```python
from build123d import *

# Parameters (mm, degrees)
EXTRUDE_1_DEPTH     = 45
SKETCH_2_W          = 70
SKETCH_2_H          = 80
EXTRUDE_2_DEPTH     = 30
SKETCH_3_W          = 70
SKETCH_3_H          = 60
CUT_EXTRUDE_1_DEPTH = 20
SKETCH_4_W          = 10
SKETCH_4_H          = 20
EXTRUDE_4_DEPTH     = 48
CUT_EXTRUDE_2_DEPTH = 125.222582488
CUT_EXTRUDE_3_DEPTH = 118.153745139


with BuildPart() as part:
    # 草圖1 → 填料-伸長1 (new body)
    with BuildSketch(Plane.XY):
        with BuildLine():
            Line((-15, 0), (-55, 0))
            Line((-55, 0), (-55, -10))
            Line((-55, -10), (-10, -10))
            Line((-10, -10), (-10, 0))
            ThreePointArc((-10, 0), (0, 10), (10, 0))
            Line((10, 0), (10, -10))
            Line((10, -10), (15, -10))
            Line((15, -10), (15, 0))
            ThreePointArc((15, 0), (0, 15), (-15, 0))
        make_face()
    extrude(amount=-EXTRUDE_1_DEPTH)

    # 草圖2 → 填料-伸長2 (add)
    with BuildSketch(Plane.ZY.offset(55)):
        with Locations((-22.5, 30)):
            Rectangle(SKETCH_2_W, SKETCH_2_H)
    extrude(amount=EXTRUDE_2_DEPTH)

    # 草圖3 → 除料-伸長1 (cut)
    with BuildSketch(Plane.ZY.offset(85)):
        with Locations((-22.5, 20)):
            Rectangle(SKETCH_3_W, SKETCH_3_H)
    extrude(amount=-CUT_EXTRUDE_1_DEPTH, mode=Mode.SUBTRACT)

    # 草圖4 → 填料-伸長4 (add)
    with BuildSketch(Plane(origin=(-55, 0, 0), x_dir=(0, 0, -1), z_dir=(1, 0, 0))):
        with Locations((22.5, 10)):
            Rectangle(SKETCH_4_W, SKETCH_4_H)
    extrude(amount=EXTRUDE_4_DEPTH)

    # 草圖6 → 除料-伸長2 (cut, through all)
    with BuildSketch(Plane.XY):
        with BuildLine():
            Line((10, 0), (10, -10))
            Line((10, -10), (-10, -10))
            Line((-10, -10), (-10, 0))
            ThreePointArc((-10, 0), (0, 10), (10, 0))
        make_face()
    extrude(amount=-CUT_EXTRUDE_2_DEPTH, mode=Mode.SUBTRACT)

    # 草圖7 → 除料-伸長3 (cut, through all)
    with BuildSketch(Plane.XY.offset(-17.5)):
        Polygon((-7, 13.266499161), (-55, 20), (-7, 20), align=None)
    extrude(amount=-CUT_EXTRUDE_3_DEPTH, mode=Mode.SUBTRACT)


solid = part.part
```
CAD build for the part. Positions are in the model's coordinates, mm. A direction names the side the tool comes from. Round coordinates to 2 decimals unless told otherwise and drop trailing zeros. Order: outer loops, then holes, each group sorted by start corner. A loop starts at its lowest first (then second) coordinate and runs counter-clockwise, first axis right, second up.
Q1. Which spindle directions (+Z, -Z, +X, -X, +Y, -Y) get a long thin tool onto all of the face, cutting with end or side? Do faces 1 (the cylindrical face through (0, 15, -22)), 2 (the flat face through (-20, -3, -45)), 3 (the flat face through (-75, 50, -23)), 4 (the flat face through (-35, 0, -9)). Say none if no direction does.
Q2. Two-plate mould, pull along X, no slides. Class faces 5 (the cylindrical face through (0, 10, -22)), 6 (the flat face through (15, -5, -22)), 7 (the flat face through (-70, 70, -23)): pulls with the +X half, pulls with the -X half, needs draft (parallel to the pull), parting line crosses it, or undercut.
Q3. Wall check: L1, parallel to X at y = -3.5, z = -39; L2, parallel to Y at x = -68, z = -28; L3, parallel to Y at x = -34, z = -31. Give the ranges that are in metal, low to high.
Q4. Drop flat-ended pins along their axis: pin 1 (6 mm diameter, centred on x = -74, z = -18.5, fed in from -Y); pin 2 (5 mm diameter, centred on y = 22.5, z = -29, fed in from -X); pin 3 (10 mm diameter, centred on x = -25.5, y = 7, fed in from -Z). Give the stop position or say it passes through.
Q5. Slice it at C-C (x = -76.5). Write the cut outline in (y, z), and give its area (3 significant figures).
Q6. Slice it at D-D (y = 28.5). Write the cut outline in (x, z), and give its area (3 significant figures).
Q7. Slice it at B-B (z = -10). Write the cut outline in (x, y).
Q8. Slice it at A-A (y = -2). Write the cut outline in (x, z).
Results below:
1. face 1: +Y
1. face 2: -Z, +X, +Y, -Y
1. face 3: +Z, -Z, -X, -Y
1. face 4: +Z, +Y
2. face 5: undercut
2. face 6: pulls with the +X half
2. face 7: needs draft
3. L1: x = -65 to -10, 10 to 15
3. L2: y = 50 to 70
3. L3: y = -10 to 0
4. pin 1: stops at y = 50
4. pin 2: stops at x = -65
4. pin 3: stops at z = -27.5
5. outline: (50, -57.5) - (70, -57.5) - (70, 12.5) - (50, 12.5) - close
5. area: 1,400 mm2
6. outline: (-65, -57.5) - (-55, -57.5) - (-55, 12.5) - (-65, 12.5) - close
6. area: 700 mm2
7. outline: (-85, 50) - (-65, 50) - (-65, -10) - (-10, -10) - (-10, 0) arc R10 cw to (10, 0) - (10, -10) - (15, -10) - (15, 0) arc R15 ccw to (-15, 0) - (-55, 0) - (-55, 70) - (-85, 70) - close
8. outline: (-65, -57.5) - (-55, -57.5) - (-55, -45) - (-10, -45) - (-10, 0) - (-55, 0) - (-55, 12.5) - (-65, 12.5) - close; (10, -45) - (15, -45) - (15, 0) - (10, 0) - close
